Input: part model. Units: mm. Frame: model coordinates. Coordinates: 2 decimals unless noted, no trailing zeros. Order: outer loops, then holes, each group sorted by start corner. A loop starts at its lowest first (then second) coordinate and runs counter-clockwise, first axis right, second up. Notation, with made-up numbers: (-39.75, 82.25) - (-26.75, 82.25) arc R16 ccw to (-26.75, 88.25) - close; hole circle Ø9 at (14, -27). An arc over 180 degrees is marked (long way). Use a Markdown table: item, result. Add a question column.
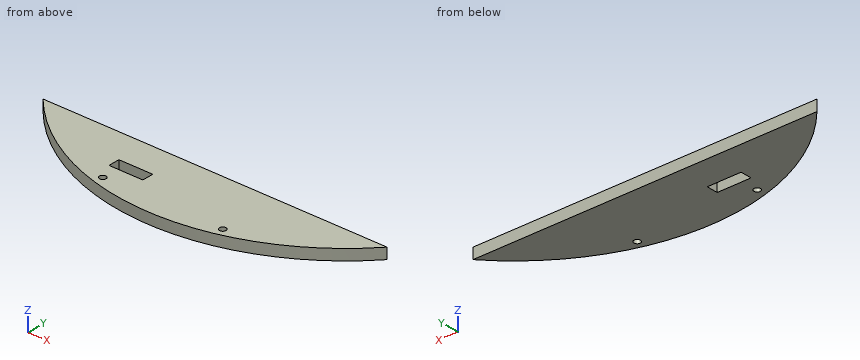
from build123d import *

# Parameters (mm, degrees)
ESQUISSE1_W             = 15.5
ESQUISSE1_H             = 5.25
BOSS_EXTRU_1_DEPTH      = 5
ESQUISSE2_R             = 1.5
ENL_V_MAT_EXTRU_1_DEPTH = 5


with BuildPart() as part:
    # Esquisse1 → Boss.-Extru.1 (new body)
    with BuildSketch(Plane.XY):
        with BuildLine():
            Line((78.965631611, -69.557615642), (-78.655820549, -69.557615642))
            ThreePointArc((-78.655820549, -69.557615642), (0.154905531, -105.175561372), (78.965631611, -69.557615642))
        make_face()
        with Locations((-23.37664966, -86.932615642)):
            Rectangle(ESQUISSE1_W, ESQUISSE1_H, mode=Mode.SUBTRACT)
    extrude(amount=BOSS_EXTRU_1_DEPTH)

    # Esquisse2 → Enlèv. mat.-Extru.1 (cut)
    with BuildSketch(Plane.XY.offset(5)):
        with Locations((-27.279170889, -97.307615642)):
            Circle(ESQUISSE2_R)
        with Locations((27.720829111, -97.307615642)):
            Circle(ESQUISSE2_R)
    extrude(amount=-ENL_V_MAT_EXTRU_1_DEPTH, mode=Mode.SUBTRACT)


solid = part.part
1) Contact query for flat-ended pins moving along their axis: P1, Ø2.5, axis at y = -86, z = 3, coming from the -X side; P2, Ø1, axis at y = -84, z = 0.5, coming from the +X side; P3, Ø8, axis at x = -58, y = -96.5, coming from the +Z side; P4, Ø1.5, axis at x = -59, z = 1.5, coming from the -Y side. Output: stop coordinate, or through.
2) Material intervals for L1, parallel to Y at x = -26, z = 3.9; L2, parallel to X at y = -88, z = 3.65; L3, parallel to Y at x = -20.5, z = 2.2, sorted ascending.
3) Cut plane B-B (z = 2.45). Return the cut outline in (x, y).
4) Cut plane D-D (x = -43). Return the cut outline in (y, z), and give its area (3 significant figures).
5) Cut plane A-A (x = -21). Return the cut outline in (y, z), and give its area (3 significant figures).
6) Cut plane C-C (y = -76). Return the cut outline in (x, z), and give its area (3 significant figures).
Computed:
| question | item | result |
|---|---|---|
| 1 | P1 | stops at x = -62.07 |
| 1 | P2 | stops at x = 64.05 |
| 1 | P3 | passes through |
| 1 | P4 | stops at y = -87.43 |
| 2 | L1 | y = -101.87 to -98.09, -96.52 to -89.56, -84.31 to -69.56 |
| 2 | L2 | x = -57.39 to -31.13, -15.63 to 57.7 |
| 2 | L3 | y = -103.12 to -89.56, -84.31 to -69.56 |
| 3 | outline | (-78.66, -69.56) arc R105 ccw to (78.97, -69.56) - close; hole (-31.13, -89.56) - (-15.63, -89.56) - (-15.63, -84.31) - (-31.13, -84.31) - close; hole circle Ø3 at (-27.28, -97.31); hole circle Ø3 at (27.72, -97.31) |
| 4 | outline | (-95.9, 0) - (-69.56, 0) - (-69.56, 5) - (-95.9, 5) - close |
| 4 | area | 132 mm2 |
| 5 | outline | (-103.02, 0) - (-89.56, 0) - (-89.56, 5) - (-103.02, 5) - close; (-84.31, 0) - (-69.56, 0) - (-69.56, 5) - (-84.31, 5) - close |
| 5 | area | 141 mm2 |
| 6 | outline | (-72.48, 0) - (72.79, 0) - (72.79, 5) - (-72.48, 5) - close |
| 6 | area | 726 mm2 |
